from build123d import *

# Parameters (mm, degrees)
F1_DEPTH    = 8
F2_R        = 1.7
F3_DEPTH    = 9.351
F2_R_2      = 2.75
F4_DEPTH    = 1.2
F5_T1_DEPTH = 14.9408405207
F5_T3_DEPTH = 18
F5_T5_DEPTH = 18


# Not quite as in the source:
# - a fillet or chamfer that OpenCascade refuses, or shapes differently, is made with other operations: its cross-section is extruded or revolved along the edge and cut away or added


with BuildPart() as f1:
    # F0 (on Top) → F1 (new body)
    with BuildSketch(Plane.XY):
        with BuildLine():
            Line((-1.5, -4.6122120506), (-1.5, -2.655654345))
            ThreePointArc((-1.5, -2.655654345), (-2.022599329, -2.2828911394), (-2.4556058316, -1.8090052515))
            Line((-2.4556058316, -1.8090052515), (-4.5, -1.8090052515))
            ThreePointArc((-4.5, -1.8090052515), (-3.3112674446, -3.5437279679), (-1.5, -4.6122120506))
        make_face()
        with BuildLine():
            ThreePointArc((2.4556058316, -1.8090052515), (2.022599329, -2.2828911394), (1.5, -2.655654345))
            Line((1.5, -2.655654345), (1.5, -4.6122120506))
            ThreePointArc((1.5, -4.6122120506), (3.3112674446, -3.5437279679), (4.5, -1.8090052515))
            Line((4.5, -1.8090052515), (2.4556058316, -1.8090052515))
        make_face()
        with BuildLine():
            ThreePointArc((4.5, -1.8090052515), (3.3112674446, -3.5437279679), (1.5, -4.6122120506))
            Line((1.5, -4.6122120506), (1.5, -9.0090052515))
            Line((1.5, -9.0090052515), (4.5, -9.0090052515))
            Line((4.5, -9.0090052515), (4.5, -1.8090052515))
        make_face()
        with BuildLine():
            Line((-1.5, -9.0090052515), (-1.5, -4.6122120506))
            ThreePointArc((-1.5, -4.6122120506), (-3.3112674446, -3.5437279679), (-4.5, -1.8090052515))
            Line((-4.5, -1.8090052515), (-4.5, -9.0090052515))
            Line((-4.5, -9.0090052515), (-1.5, -9.0090052515))
        make_face()
        with BuildLine():
            Line((-4.5, -1.8090052515), (-2.4556058316, -1.8090052515))
            ThreePointArc((-2.4556058316, -1.8090052515), (-0.9520772589, 2.8975936384), (3.05, 0))
            ThreePointArc((3.05, 0), (2.8975936384, -0.9520772589), (2.4556058316, -1.8090052515))
            Line((2.4556058316, -1.8090052515), (4.5, -1.8090052515))
            ThreePointArc((4.5, -1.8090052515), (4.7616961264, -0.9212762886), (4.85, 0))
            ThreePointArc((4.85, 0), (-0.9212762886, 4.7616961264), (-4.5, -1.8090052515))
        make_face()
    extrude(amount=F1_DEPTH)

    # F2 (on face) → F3 (cut, through all)
    with BuildSketch(Plane.YZ.offset(4.5)):
        with Locations((-5.6298957206, 4)):
            Circle(F2_R)
    extrude(amount=-F3_DEPTH, mode=Mode.SUBTRACT)

    # F2 (on face) → F4 (cut)
    with BuildSketch(Plane.YZ.offset(4.5)):
        Polygon((-8.4798957206, 5.6454482672), (-8.4798957206, 2.3545517328), (-5.6298957206, 0.7091034656), (-2.7798957206, 2.3545517328), (-2.7798957206, 5.6454482672), (-5.6298957206, 7.2908965344), align=None)
        with Locations((-5.6298957206, 4)):
            Circle(F2_R_2, mode=Mode.SUBTRACT)
        with Locations((-5.6298957206, 4)):
            Circle(F2_R_2)
        with Locations((-5.6298957206, 4)):
            Circle(F2_R, mode=Mode.SUBTRACT)
    extrude(amount=-F4_DEPTH, mode=Mode.SUBTRACT)

    # F5: fillet of radius 3 on 6 edges, made by hand

    # F5_s2 → F5_t1 (cut)
    with BuildSketch(Plane.XY.offset(-3.4704202604)):
        with BuildLine():
            ThreePointArc((2.2685950413, -2.0386212347), (1.6987311022, -2.9700941027), (1.5, -4.0438224491))
            Line((1.5, -4.0438224491), (1.5, -2.655654345))
            ThreePointArc((1.5, -2.655654345), (1.9093872345, -2.3783902936), (2.2685950413, -2.0386212347))
        make_face()
        with BuildLine():
            ThreePointArc((-1.5, -4.0438224491), (-1.6987311022, -2.9700941027), (-2.2685950413, -2.0386212347))
            ThreePointArc((-2.2685950413, -2.0386212347), (-1.9093872345, -2.3783902936), (-1.5, -2.655654345))
            Line((-1.5, -2.655654345), (-1.5, -4.0438224491))
        make_face()
    extrude(amount=F5_T1_DEPTH, mode=Mode.SUBTRACT)

    # F5_s4 → F5_t3 (cut)
    with BuildSketch(Plane.YZ.offset(-6)):
        with BuildLine():
            ThreePointArc((-6.0090052515, 8), (-8.1303255951, 7.1213203436), (-9.0090052515, 5))
            Line((-9.0090052515, 5), (-9.0090052515, 8))
            Line((-9.0090052515, 8), (-6.0090052515, 8))
        make_face()
        with BuildLine():
            ThreePointArc((-6.0090052515, 0), (-8.1303255951, 0.8786796564), (-9.0090052515, 3))
            Line((-9.0090052515, 3), (-9.0090052515, 0))
            Line((-9.0090052515, 0), (-6.0090052515, 0))
        make_face()
    extrude(amount=F5_T3_DEPTH, mode=Mode.SUBTRACT)

    # F5_s6 → F5_t5 (cut)
    with BuildSketch(Plane.YZ.offset(-12)):
        with BuildLine():
            ThreePointArc((-6.0090052515, 8), (-8.1303255951, 7.1213203436), (-9.0090052515, 5))
            Line((-9.0090052515, 5), (-9.0090052515, 8))
            Line((-9.0090052515, 8), (-6.0090052515, 8))
        make_face()
        with BuildLine():
            ThreePointArc((-6.0090052515, 0), (-8.1303255951, 0.8786796564), (-9.0090052515, 3))
            Line((-9.0090052515, 3), (-9.0090052515, 0))
            Line((-9.0090052515, 0), (-6.0090052515, 0))
        make_face()
    extrude(amount=F5_T5_DEPTH, mode=Mode.SUBTRACT)


solid = f1.part
Work out the finished part from the listing and answer in its coordinate system (mm). A direction names the side the tool comes from. Round coordinates to 2 decimals unless told otherwise and drop trailing zeros. Write each loop counter-clockwise with the first axis right and the second up, starting at its lowest first coordinate (ties: lowest second). Pieces come first, ordered by that corner, then holes. Notation, with made-up numbers: (21, 9.5) - (54, 9.5) arc R14 ccw to (54, 22.5) - close; hole circle Ø9 at (41, -31.75). An arc over 180 degrees is marked (long way). Answer in a Markdown table with one row per item. Add a question column.
1. Given pin 1 (3.5 mm diameter, centred on y = -4, z = 6, fed in from -X); pin 2 (2.5 mm diameter, centred on y = -7, z = 4, fed in from +X), each flat-ended and moving along its own axis, determine where each tip first touches the part or whether it passes through.
2. Find the intervals of material crossed by line 1 along Y through (x, z) = (-2.7, 4); line 2 along Y through (x, z) = (0, 3.25); line 3 along Z through (x, y) = (2.75, -5.75), in increasing order. Write a range as from..to.
3. A cutting plane is placed at B-B, the plane z = 2.75. Determine the outline of the cut face in (x, y).
4. A cutting plane is placed at A-A, the plane y = -6.25. Determine the outline of the cut face in (x, z).
5. For faces 1 (the flat face through (3.91, -7.07, 1.54)), 2 (the flat face through (4.5, -3, 2)), 3 (the cylindrical face through (1.704, -2.956, 3.944)), determine the directions among +Z, -Z, +X, -X, +Y, -Y from which every point of the face is accessible in a straight line to the end or side of a thin tool.
6. The mould has two halves that part along Y. Classify faces 4 (the flat face through (1.5, -8, 4)), 5 (the cylindrical face through (2.98, -8.11, 0.86)), 6 (the flat face through (3.9, -7, 6.5)): +Y half, -Y half, draft (parallel to the pull), parting line (faces both ways), or undercut.
7. A cutting plane is placed at D-D, the plane y = 1.5. Determine the outline of the cut face in (x, z), and give its area (3 significant figures).
8. A cutting plane is placed at C-C, the plane x = 2. Determine the outline of the cut face in (y, z), and give its area (3 significant figures).
Worked out:
| question | item | result |
|---|---|---|
| 1 | pin 1 | x = -4.5 |
| 1 | pin 2 | x = 3.3 |
| 2 | line 1 | -9.01..-7.33, -3.93..-1.42, 1.42..4.03 |
| 2 | line 2 | 3.05..4.85 |
| 2 | line 3 | 0..2.3, 5.7..8 |
| 3 | outline | (-4.5, -9) - (-1.5, -9) - (-1.5, -6.78) - (-4.5, -6.78) - close; (-4.5, -4.48) - (-1.5, -4.48) - (-1.5, -4.04) arc R3 ccw to (-2.27, -2.04) arc R3.05 cw (long way) to (2.27, -2.04) arc R3 ccw to (1.5, -4.04) - (1.5, -4.48) - (3.3, -4.48) - (3.3, -2.78) - (4.5, -2.78) - (4.5, -1.81) arc R4.85 ccw (long way) to (-4.5, -1.81) - close; (1.5, -9) - (4.5, -9) - (4.5, -8.48) - (3.3, -8.48) - (3.3, -6.78) - (1.5, -6.78) - close |
| 4 | outline | (-4.5, 0.01) - (-1.5, 0.01) - (-1.5, 2.42) - (-4.5, 2.42) - close; (-4.5, 5.58) - (-1.5, 5.58) - (-1.5, 7.99) - (-4.5, 7.99) - close; (1.5, 0.01) - (4.5, 0.01) - (4.5, 1.07) - (3.3, 1.07) - (3.3, 2.42) - (1.5, 2.42) - close; (1.5, 5.58) - (3.3, 5.58) - (3.3, 6.93) - (4.5, 6.93) - (4.5, 7.99) - (1.5, 7.99) - close |
| 5 | face 1 | +X |
| 5 | face 2 | +Z, -Z, +X, -Y |
| 5 | face 3 | +Z, -Z |
| 6 | face 4 | draft |
| 6 | face 5 | -Y half |
| 6 | face 6 | undercut |
| 7 | outline | (-4.61, 0) - (-2.66, 0) - (-2.66, 8) - (-4.61, 8) - close; (2.66, 0) - (4.61, 0) - (4.61, 8) - (2.66, 8) - close |
| 7 | area | 31.3 mm^2 |
| 8 | outline | (-9.01, 3) arc R3 ccw to (-6.01, 0) - (-2.39, 0) - (-2.39, 8) - (-6.01, 8) arc R3 ccw to (-9.01, 5) - close; (2.3, 0) - (4.42, 0) - (4.42, 8) - (2.3, 8) - close; hole circle Ø3.4 at (-5.63, 4) |
| 8 | area | 57.0 mm^2 |
